Verification items for the finished model (mm, model axes). Round coordinates to 2 decimals unless told otherwise and drop trailing zeros. Order: outer loops, then holes, each group sorted by start corner. A loop starts at its lowest first (then second) coordinate and runs counter-clockwise, first axis right, second up. Notation, with made-up numbers: (84.25, -37) -> (130.25, -37) arc R21 cw to (130.25, -25) -> close; hole circle Ø10 at (45.5, 6). An arc over 180 degrees is marked (long way). Put each result on its own line as item: value.
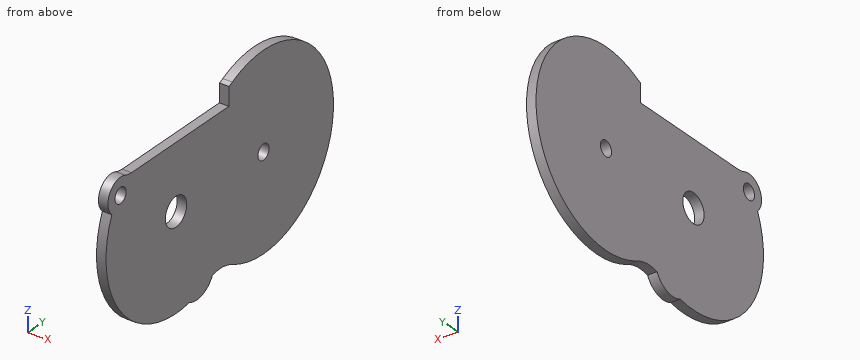
```python
from build123d import *

# Parameters (mm, degrees)
SKETCH1_R           = 1.6
SKETCH1_R_2         = 3.05
BOSS_EXTRUDE1_DEPTH = 2


with BuildPart() as part:
    # Sketch1 → Boss-Extrude1 (new body)
    with BuildSketch(Plane(origin=(-4.933780691, 0, 0), x_dir=(0, 0, -1), z_dir=(1, 0, 0))):
        with BuildLine():
            Line((8.316418793, -3.583005728), (8.316418793, -31.394980118))
            ThreePointArc((8.316418793, -31.394980118), (8.228435382, -32.328839328), (7.967581583, -33.22983289))
            ThreePointArc((7.967581583, -33.22983289), (9.37872929, -37.584960404), (13.923442901, -37.033551565))
            ThreePointArc((13.923442901, -37.033551565), (34.408956218, -34.312472042), (41.551457155, -14.920586884))
            ThreePointArc((41.551457155, -14.920586884), (41.753619834, -11.13958937), (39.247730179, -8.301045906))
            ThreePointArc((39.247730179, -8.301045906), (39.005043324, -5.412218315), (39.807804245, -2.626577156))
            ThreePointArc((39.807804245, -2.626577156), (21.911418793, 26.301994272), (4.015033341, -2.626577156))
            ThreePointArc((4.015033341, -2.626577156), (4.231547099, -3.098268174), (4.417019815, -3.583005728))
            Line((4.417019815, -3.583005728), (8.316418793, -3.583005728))
        make_face()
        with Locations((11.316418793, -34.550926886)):
            Circle(SKETCH1_R, mode=Mode.SUBTRACT)
        with Locations((21.911418793, -18.698005728)):
            Circle(SKETCH1_R_2, mode=Mode.SUBTRACT)
        with Locations((21.911418793, 6.301994272)):
            Circle(SKETCH1_R, mode=Mode.SUBTRACT)
    extrude(amount=BOSS_EXTRUDE1_DEPTH)


solid = part.part
```
Item 1: Sectioned sample at A-A, the plane y = -20. Record the boundary of the cut face in (x, z), then the cut area to 3 significant figures.
Geometry check:
outline: (-4.93, -41.87) -> (-2.93, -41.87) -> (-2.93, -24.67) -> (-4.93, -24.67) -> close; (-4.93, -19.15) -> (-2.93, -19.15) -> (-2.93, -8.32) -> (-4.93, -8.32) -> close
area: 56.1 mm2
Item 2: Sectioned sample at D-D, the plane z = -30. Record the boundary of the cut face in (x, y).
Geometry check:
outline: (-4.93, -36.99) -> (-2.93, -36.99) -> (-2.93, 24.59) -> (-4.93, 24.59) -> close
Item 3: Sectioned sample at B-B, the plane z = -22. Record the boundary of the cut face in (x, y), then the cut area to 3 significant figures.
Geometry check:
outline: (-4.93, -38.7) -> (-2.93, -38.7) -> (-2.93, -21.75) -> (-4.93, -21.75) -> close; (-4.93, -15.65) -> (-2.93, -15.65) -> (-2.93, 4.7) -> (-4.93, 4.7) -> close; (-4.93, 7.9) -> (-2.93, 7.9) -> (-2.93, 26.3) -> (-4.93, 26.3) -> close
area: 111 mm2
Item 4: Sectioned sample at C-C, the plane x = -3.85. Record the boundary of the cut face in (y, z), then the cut area to 3 significant figures.
Geometry check:
outline: (-37.03, -13.92) arc R20 ccw to (-14.92, -41.55) arc R5 ccw to (-8.3, -39.25) arc R8 cw to (-2.63, -39.81) arc R20 ccw (long way) to (-2.63, -4.02) arc R8 cw to (-3.58, -4.42) -> (-3.58, -8.32) -> (-31.39, -8.32) arc R5 cw to (-33.23, -7.97) arc R3.6 ccw to start; hole circle Ø3.2 at (-34.55, -11.32); hole circle Ø6.1 at (-18.7, -21.91); hole circle Ø3.2 at (6.3, -21.91)
area: 2,030 mm2
Item 5: Depth check by flat-ended pin: pin 1 Ø1 at (x, y) = (-4.5, -12) entering from +Z; pin 2 Ø1 at (x, z) = (-4.5, -32.5) entering from -Y; pin 3 Ø8 at (y, z) = (-18.7, -21.91) entering from +X; pin 4 Ø1 at (x, y) = (-4.5, 10) entering from -Z. Enter the tip coordinate at first touch or a pass-through.
Geometry check:
pin 1: z = -8.32
pin 2: y = -35.97
pin 3: x = -2.93
pin 4: z = -41.65
Item 6: Material ranges on line 1 along Y through (x, z) = (-4.3, -22); line 2 along Z through (x, y) = (-3.95, -34); line 3 along Z through (x, y) = (-3.35, 7), recorded low to high.
Geometry check:
line 1: -38.7 to -21.75, -15.65 to 4.7, 7.9 to 26.3
line 2: -34.79 to -12.82, -9.81 to -7.76
line 3: -41.9 to -23.35, -20.47 to -1.92
